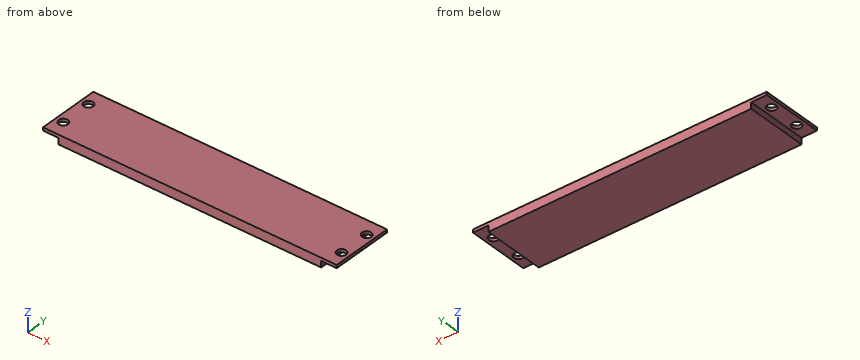
Autodesk Inventor part; units mm, degrees
ref_plane "YZ Plane" through (0, 0, 0) normal (1, 0, 0) x (0, 1, 0)
ref_plane "XZ Plane" through (0, 0, 0) normal (0, 1, 0) x (-1, 0, 0)
ref_plane "XY Plane" through (0, 0, 0) normal (0, 0, 1) x (1, 0, 0)
sketch "Эскиз1" plane through (0, 0, 0) normal (0, 0, 1) x (1, 0, 0)
  point P0 (0, 0)
sketch "Эскиз2" plane through (0, 0, 0) normal (0, 0, 1) x (1, 0, 0)
  line L0 (0, 0) -> (85, 0)
  line L1 (85, 0) -> (85, 20)
  line L2 (85, 20) -> (0, 20)
  line L3 (0, 20) -> (0, 0)
  dimension "d0" = 85
  dimension "d1" = 20
extrude "Выдавливание1" add sketch "Эскиз2" along normal blind 3
sketch "Эскиз3" plane through (0, 0, 3) normal (0, 0, 1) x (1, 0, 0)
  line L0 (0, 20) -> (0, 0)
  line L1 (85, 0) -> (85, 20)
  line L2 (0, 20) -> (-5, 20)
  line L3 (-5, 20) -> (-5, 0)
  line L4 (-5, 0) -> (0, 0)
  line L5 (0, 0) -> (0, 20)
  circle A0 centre (-2.5, 15) radius 1.5
  circle A1 centre (-2.5, 5) radius 1.5
  line L6 (85, 20) -> (85, 0)
  line L7 (85, 20) -> (90, 20)
  line L8 (90, 20) -> (90, 0)
  line L9 (90, 0) -> (85, 0)
  line L10 (85, 0) -> (85, 20)
  circle A2 centre (87.5, 15) radius 1.5
  circle A3 centre (87.5, 5) radius 1.5
  dimension "d4" = 5
  dimension "d7" = 3
  dimension "d8" = 3
extrude "Выдавливание2" add sketch "Эскиз3" against normal blind 1
properties part number "Крышка на ESC" material "Пластик ПЭТ"
Work out the finished part from the listing and answer in its coordinate system (mm). Round coordinates to 2 decimals unless told otherwise and drop trailing zeros. Write each loop counter-clockwise with the first axis right and the second up, starting at its lowest first coordinate (ties: lowest second). Pieces come first, ordered by that corner, then holes.
1) A cutting plane is placed at D-D on z = 1.4. Determine the outline of the cut face in (x, y).
2) Consider probe 1 along Y at (x, z) = (-2.5, 2.75); probe 2 along X at (y, z) = (14, 1.9). Determine where each line is inside the solid, lowest interval first.
3) A cutting plane is placed at C-C on y = 2. Determine the outline of the cut face in (x, z).
4) A cutting plane is placed at B-B on x = -2.5. Determine the outline of the cut face in (y, z).
5) A cutting plane is placed at A-A on y = 15. Determine the outline of the cut face in (x, z), and give its area (3 significant figures).
6) Flat-ended cylindrical pins translate along their axes: P1, Ø2.5, axis at x = -2.5, y = 5, coming from the -Z side; P2, Ø1.5, axis at x = -1.5, y = 11, coming from the -Z side; P3, Ø1.6, axis at y = 9, z = 1, coming from the -X side; P4, Ø1, axis at y = 12, z = 0.5, coming from the +X side. Find the tip coordinate at first contact, or state that the pin passes through.
Entries:
1. outline: (0, 0) - (85, 0) - (85, 20) - (0, 20) - close
2. probe 1: y = 0 to 3.5, 6.5 to 13.5, 16.5 to 20
2. probe 2: x = 0 to 85
3. outline: (-5, 2) - (0, 2) - (0, 0) - (85, 0) - (85, 2) - (90, 2) - (90, 3) - (-5, 3) - close
4. outline: (0, 2) - (3.5, 2) - (3.5, 3) - (0, 3) - close; (6.5, 2) - (13.5, 2) - (13.5, 3) - (6.5, 3) - close; (16.5, 2) - (20, 2) - (20, 3) - (16.5, 3) - close
5. outline: (-5, 2) - (-4, 2) - (-4, 3) - (-5, 3) - close; (-1, 2) - (0, 2) - (0, 0) - (85, 0) - (85, 2) - (86, 2) - (86, 3) - (-1, 3) - close; (89, 2) - (90, 2) - (90, 3) - (89, 3) - close
5. area: 259 mm2
6. P1: passes through
6. P2: stops at z = 2
6. P3: stops at x = 0
6. P4: stops at x = 85
